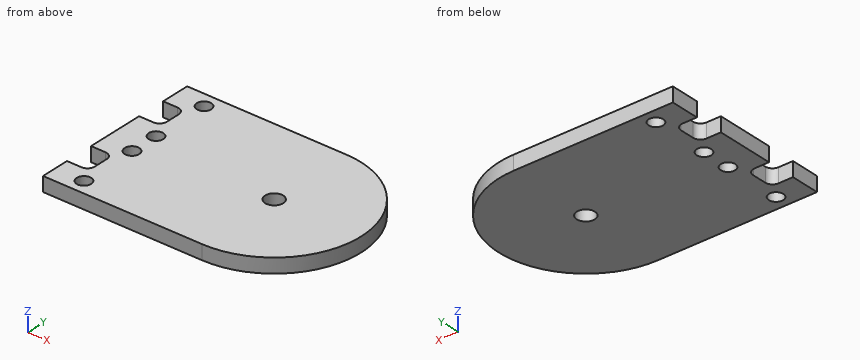
from build123d import *

# Parameters (mm, degrees)
SKETCH_1_R      = 1.25
SKETCH_1_R_2    = 1
EXTRUDE_1_DEPTH = 2


with BuildPart() as part:
    # 草圖1 → 填料-伸長1 (new body)
    with BuildSketch(Plane.XY):
        with BuildLine():
            Line((-38.093061493, 13.879025542), (-16.093061493, 13.879025542))
            ThreePointArc((-16.093061493, 13.879025542), (-4.093061493, 1.879025542), (-16.093061493, -10.120974458))
            Line((-16.093061493, -10.120974458), (-38.093061493, -10.120974458))
            Line((-38.093061493, -10.120974458), (-38.093061493, -6.120974458))
            Line((-38.093061493, -6.120974458), (-36.093061493, -6.120974458))
            ThreePointArc((-36.093061493, -6.120974458), (-35.385954712, -5.828081239), (-35.093061493, -5.120974458))
            Line((-35.093061493, -5.120974458), (-35.093061493, -3.120974458))
            ThreePointArc((-35.093061493, -3.120974458), (-35.385954712, -2.413867677), (-36.093061493, -2.120974458))
            Line((-36.093061493, -2.120974458), (-38.093061493, -2.120974458))
            Line((-38.093061493, -2.120974458), (-38.093061493, 5.879025542))
            Line((-38.093061493, 5.879025542), (-36.093061493, 5.879025542))
            ThreePointArc((-36.093061493, 5.879025542), (-35.385954712, 6.171918761), (-35.093061493, 6.879025542))
            Line((-35.093061493, 6.879025542), (-35.093061493, 8.879025542))
            ThreePointArc((-35.093061493, 8.879025542), (-35.385954712, 9.586132323), (-36.093061493, 9.879025542))
            Line((-36.093061493, 9.879025542), (-38.093061493, 9.879025542))
            Line((-38.093061493, 9.879025542), (-38.093061493, 13.879025542))
        make_face()
        with Locations((-16.093061493, 1.879025542)):
            Circle(SKETCH_1_R, mode=Mode.SUBTRACT)
        with Locations((-34.093061493, 11.879025542)):
            Circle(SKETCH_1_R_2, mode=Mode.SUBTRACT)
        with Locations((-34.093061493, 3.879025542)):
            Circle(SKETCH_1_R_2, mode=Mode.SUBTRACT)
        with Locations((-34.093061493, -8.120974458)):
            Circle(SKETCH_1_R_2, mode=Mode.SUBTRACT)
        with Locations((-34.093061493, -0.120974458)):
            Circle(SKETCH_1_R_2, mode=Mode.SUBTRACT)
    extrude(amount=EXTRUDE_1_DEPTH)


solid = part.part
For this review, take the finished solid that the model builds, in its own axes (mm). Round coordinates to 2 decimals unless told otherwise and drop trailing zeros. Order: outer loops, then holes, each group sorted by start corner. A loop starts at its lowest first (then second) coordinate and runs counter-clockwise, first axis right, second up. Notation, with made-up numbers: M 71.25,-5 L 116.25,-5 A17 cw 116.25,2 Z; hole C 15.5,-40 d2. An arc over 180 degrees is marked long. Write each question's results on one line, items separated by ' | '. Start each with the question number.
1. To check wall thickness, follow L1, parallel to Y at x = -34, z = 0.45; L2, parallel to Y at x = -16, z = 1.7; L3, parallel to Y at x = -17, z = 0.65. State the ranges of each line that lie inside material, in increasing order. Write a range as [from, to].
2. Add section B-B (y = 1.25). State the section outline as (x, z) points.
3. Add section D-D (x = -11.5). State the section outline as (y, z) points, then the cut area to 3 significant figures.
4. Add section C-C (z = 1.5). State the section outline as (x, y) points, then the cut area to 3 significant figures.
5. Add section A-A (x = -17). State the section outline as (y, z) points, then the cut area to 3 significant figures.
6. Clearance check with a flat-ended pin moving along its axis: pin 1 Ø0.6 at (y, z) = (-4.5, 1) entering from -X. State where the tip first meets the part, or that it passes through.
Output values:
1) L1: [-10.12, -9.12], [-7.13, -1.12], [0.87, 2.88], [4.87, 10.88], [12.87, 13.88] | L2: [-10.12, 0.63], [3.13, 13.88] | L3: [-10.12, 1.02], [2.74, 13.88]
2) outline: M -38.09,0 L -17.17,0 L -17.17,2 L -38.09,2 Z; M -15.01,0 L -4.11,0 L -4.11,2 L -15.01,2 Z
3) outline: M -9.21,0 L 12.97,0 L 12.97,2 L -9.21,2 Z | area: 44.3 mm^2
4) outline: M -38.09,-10.12 L -16.09,-10.12 A12 ccw -16.09,13.88 L -38.09,13.88 L -38.09,9.88 L -36.09,9.88 A1 cw -35.09,8.88 L -35.09,6.88 A1 cw -36.09,5.88 L -38.09,5.88 L -38.09,-2.12 L -36.09,-2.12 A1 cw -35.09,-3.12 L -35.09,-5.12 A1 cw -36.09,-6.12 L -38.09,-6.12 Z; hole C -34.09,-8.12 d2; hole C -34.09,-0.12 d2; hole C -34.09,3.88 d2; hole C -34.09,11.88 d2; hole C -16.09,1.88 d2.5 | area: 714 mm^2
5) outline: M -10.12,0 L 1.02,0 L 1.02,2 L -10.12,2 Z; M 2.74,0 L 13.88,0 L 13.88,2 L 2.74,2 Z | area: 44.6 mm^2
6) pin 1: x = -35.09
